Autodesk Inventor part; units mm, degrees
ref_plane "YZ Plane" through (0, 0, 0) normal (1, 0, 0) x (0, 1, 0)
ref_plane "XZ Plane" through (0, 0, 0) normal (0, 1, 0) x (-1, 0, 0)
ref_plane "XY Plane" through (0, 0, 0) normal (0, 0, 1) x (1, 0, 0)
sketch "Szkic1" plane through (0, 0, 0) normal (0, 0, 1) x (1, 0, 0)
  line L0 (0, 7.75) -> (46, 7.75)
  line L1 (46, 7.75) -> (46, -7.75)
  line L2 (46, -7.75) -> (42.75, -7.75)
  line L3 (0, -7.75) -> (0, 7.75)
  line L4 (33.25, -7.75) -> (0, -7.75)
  arc A0 (42.75, -7.75) -> (33.25, -7.75) centre (38, -7.75) ccw
  line L5 (0, -10.85) -> (0, 10.85)
  line L6 (0, -7.75) -> (33.25, -7.75)
  line L7 (42.75, -7.75) -> (46, -7.75)
  point P0 (0, 0)
  point P1 (0, 0)
  dimension "d0" = 46
  dimension "d1" = 15.5
  dimension "d9" = 38
  dimension "d10" = 4.75
  dimension "d11" = 0
revolve "Obrót1" add sketch "Szkic1" angle 360 about axis through (0, -10, 0) along (0, 1, 0)
sketch "Szkic2" plane through (0, -7.75, 0) normal (0, -1, 0) x (1, 0, 0)
  arc A0 (1.3565, -2.1) -> (-1.3565, -2.1) centre (0, 0) ccw
  line L0 (1.3565, -2.1) -> (-1.3565, -2.1)
  point P0 (0, -2.1)
  point P1 (0, 2.5)
  dimension "d5" = 5
  dimension "d15" = 4.6
extrude "Wyciągnięcie proste1" cut sketch "Szkic2" against normal blind 13.5
chamfer "Faza1" distance 0.5 angle 45 2 edges at (-42.75, -7.75, 0) (-33.25, -7.75, 0)
sketch "Szkic3" plane through (0, 7.75, 0) normal (0, 1, 0) x (1, 0, 0)
  circle A0 centre (-17.5, -9.75) radius 1.5
  line L0 (64.4, 0) -> (-64.4, 0)
  line L1 (0, 64.4) -> (0, -64.4)
  circle A1 centre (-17.5, 9.75) radius 1.5
  circle A2 centre (17.5, -9.75) radius 1.5
  circle A3 centre (17.5, 9.75) radius 1.5
  point P0 (0, 0)
  dimension "d16" = 3
  dimension "d17" = 9.75
  dimension "d18" = 17.5
extrude "Wyciągnięcie proste2" cut sketch "Szkic3" against normal blind 7
properties part number "Base_arm_mount"
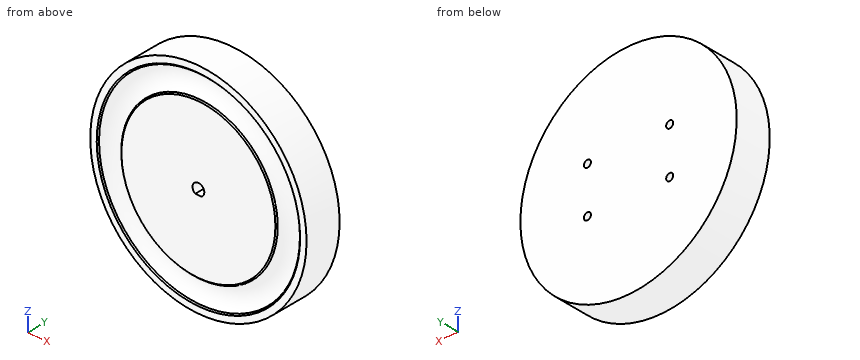
The listing builds one solid part. Answer for the finished solid, in the listing's coordinates (mm). Round coordinates to 2 decimals unless told otherwise and drop trailing zeros. Write each loop counter-clockwise with the first axis right and the second up, starting at its lowest first coordinate (ties: lowest second). Pieces come first, ordered by that corner, then holes. Notation, with made-up numbers: (48, -3.75) -> (65, -3.75) arc R25 cw to (65, 34.25) -> close; hole circle Ø11 at (43.5, -16.5). An arc over 180 degrees is marked (long way). Use CSV: the item, a comma, the result in double quotes. Start each with the question number.
(1) Each of these flat-tipped pins is pushed along its axis until it touches: pin 1 (3 mm diameter, centred on y = 4.5, z = 6.5, fed in from +X); pin 2 (2 mm diameter, centred on x = -0.5, y = -3, fed in from +Z); pin 3 (2.5 mm diameter, centred on x = -17.5, z = 9.75, fed in from +Y). Where does it stop, or does it pass through?
(2) Consider L1, parallel to X at y = -5.5, z = -21.5; L2, parallel to X at y = -4.5, z = 0; L3, parallel to X at y = 6, z = -9.75. Determine where each line is inside the solid, lowest interval first. Write a range as from..to.
(3) Section A-A on y = -6 is taken. Give the vertices of the cut face in (x, z).
A:
1,pin 1,"stops at x = 45.73"
1,pin 2,"stops at z = 46"
1,pin 3,"stops at y = 0.75"
2,L1,"x = -40.67..-36.29, -26.1..26.1, 36.29..40.67"
2,L2,"x = -46..-41.46, -34.54..-2.5, 2.5..34.54, 41.46..46"
2,L3,"x = -44.95..-19, -16..16, 19..44.95"
3,outline,"circle Ø92 at (0, 0); circle Ø67.17 at (0, 0); hole circle Ø84.83 at (0, 0); hole (-1.36, -2.1) -> (1.36, -2.1) arc R2.5 ccw (long way) to start"
